For this review, take the finished solid that the model builds, in its own axes (mm). A direction names the side the tool comes from. Coordinates: 2 decimals unless noted, no trailing zeros. Loops run counter-clockwise (first coordinate to the right, second up) from the corner with the lowest first, then second, coordinate; pieces in that order, holes last. Notation, with made-up numbers: (12, 65.25) - (51, 65.25) arc R19 cw to (51, 69.25) - close; hole circle Ø7 at (19.5, -17). An arc over 180 degrees is marked (long way). Answer as a JSON object with one key per item and string values. Group by question number.
Item 1: We need section C-C (x = 3.25). Give the boundary of the cut face in (y, z).
Item 2: We need section A-A (x = -4.5). Give the boundary of the cut face in (y, z).
Item 3: Mouldability with a two-part tool opening along Z and no side actions: class faces 4 (the cylindrical face through (0.01, -7.985, -5.301)), 5 (the flat face through (-4, -2, -5)), 6 (the flat face through (-4, -6, 3)), 7 (the flat face through (0, -5, -2)) as released by +Z, released by -Z, zero draft, split by the parting line, or undercut.
Item 4: We need section B-B (y = 2.5). Give the boundary of the cut face in (x, z).
Item 5: Clearance check with flat-ended pins moving along their axes: pin 1 (6 mm diameter, centred on x = -2.5, z = -1.5, fed in from -Y); pin 2 (1.2 mm diameter, centred on x = -4, y = -7.5, fed in from +Z); pin 3 (1.3 mm diameter, centred on y = 0, z = 5, fed in from -X); pin 4 (1.5 mm diameter, centred on x = 3.5, z = 4, fed in from -Y). State where each tip first meets the part, or that it passes through.
Item 6: To check wall thickness, follow line 1 (Y direction, x = -5, z = 0.5); line 2 (X direction, y = -2.5, z = 4.25); line 3 (Z direction, x = 5.5, y = 2.75). State the ranges of each line that lie inside material, in increasing order.
Item 7: Tool access review of faces 1 (the cylindrical face through (-4.077, -10.416, -0.314)), 2 (the conical face through (-0.297, -0.904, 4.867)), 3 (the flat face through (4, -6, 3)): name each direction out of +Z, -Z, +X, -X, +Y, -Y from which nothing blocks a thin tool from reaching the whole face with its end or side.
from build123d import *

# Parameters (mm, degrees)
BOSS_EXTRUDE1_DEPTH      = 5
CUT_EXTRUDE8_DEPTH       = 10.848857802
CUT_EXTRUDE8_DEPTH_BACK  = 10.848857802
REVOLVE1_ANGLE           = 180
SKETCH24_W               = 3.9
SKETCH24_H               = 6
BOSS_EXTRUDE2_DEPTH      = 4
SKETCH25_W               = 3.9
SKETCH25_H               = 3
REVOLVE2_ANGLE           = 180
SKETCH26_R               = 1.45
CUT_EXTRUDE9_DEPTH       = 19
BOSS_EXTRUDE4_DEPTH      = 3.7
CUT_EXTRUDE10_DEPTH      = 19
CUT_EXTRUDE10_DEPTH_BACK = 19


with BuildPart() as part:
    # Sketch2 → Boss-Extrude1 (new, symmetric)
    with BuildSketch(Plane(origin=(0, 0, 0), x_dir=(1, 0, 0), z_dir=(0, 1, 0))):
        Polygon((-3, 6), (3, 6), (6, 3), (6, -3), (3, -6), (-3, -6), (-6, -3), (-6, 3), align=None)
    extrude(amount=BOSS_EXTRUDE1_DEPTH, both=True)

    # Sketch22 → Cut-Extrude8 (cut, two sides: drawn at the far end of the back side and taken through both)
    with BuildSketch(Plane(origin=(0, 0, 0), x_dir=(0, 0, -1), z_dir=(1, 0, 0)).offset(-CUT_EXTRUDE8_DEPTH_BACK)):
        Polygon((0, -5), (-6, -5), (-6, -1.535898385), align=None)
    extrude(amount=CUT_EXTRUDE8_DEPTH + CUT_EXTRUDE8_DEPTH_BACK, mode=Mode.SUBTRACT)

    # Sketch23 → Revolve1 (revolve)
    with BuildSketch(Plane(origin=(0, 5, 0), x_dir=(1, 0, 0), z_dir=(0, 1, 0))):
        Polygon((-6, 0), (-6, 3), (-3, 6), (3, 6), (6, 3), (6, 0), align=None)
    revolve(axis=Axis((6, 5, 0), (1, 0, 0)), revolution_arc=REVOLVE1_ANGLE)

    # Sketch24 → Boss-Extrude2 (add, symmetric)
    with BuildSketch(Plane.XZ.offset(5)):
        with Locations((-4.05, 0)):
            Rectangle(SKETCH24_W, SKETCH24_H)
    boss_extrude2 = extrude(amount=BOSS_EXTRUDE2_DEPTH, both=True)

    # Sketch25 → Revolve2 (revolve)
    with BuildSketch(Plane.XZ.offset(9)):
        with Locations((-4.05, 1.5)):
            Rectangle(SKETCH25_W, SKETCH25_H)
    revolve2 = revolve(axis=Axis((-6, -9, 0), (1, 0, 0)), revolution_arc=REVOLVE2_ANGLE)

    # Sketch26 → Cut-Extrude9 (cut, symmetric)
    with BuildSketch(Plane.ZY.offset(6)):
        with Locations((0, -9)):
            Circle(SKETCH26_R)
    cut_extrude9 = extrude(amount=CUT_EXTRUDE9_DEPTH, both=True, mode=Mode.SUBTRACT)

    # Mirror1: Boss-Extrude2, Revolve2, Cut-Extrude9 across plane
    add(boss_extrude2.mirror(Plane(origin=(0, 0, 0), x_dir=(0, 0, 1), z_dir=(1, 0, 0))))
    add(revolve2.mirror(Plane(origin=(0, 0, 0), x_dir=(0, 0, 1), z_dir=(1, 0, 0))))
    add(cut_extrude9.mirror(Plane(origin=(0, 0, 0), x_dir=(0, 0, 1), z_dir=(1, 0, 0))), mode=Mode.SUBTRACT)

    # Sketch30 → Cut-Revolve1 (revolve, cut)
    with BuildSketch(Plane(origin=(0, -3.75, 2.165063509), x_dir=(1, 0, 0), z_dir=(0, -0.8660254037844418, 0.49999999999999484))):
        Polygon((0, 3.42820323), (-0.75, 2.67820323), (-0.75, 1.92820323), (0.75, 1.92820323), (0.75, 2.67820323), align=None)
    revolve(axis=Axis((-6, -1.535898385, 6), (1, 0, 0)), mode=Mode.SUBTRACT)

    # Sketch34 → Boss-Extrude4 (add)
    with BuildSketch(Plane.XZ.offset(5)):
        Polygon((-6, -3), (-2.1, -3), (2.1, -3), (6, -3), (3, -6), (-3, -6), align=None)
    extrude(amount=BOSS_EXTRUDE4_DEPTH)

    # Sketch35 → Cut-Revolve3 (revolve, cut)
    with BuildSketch(Plane.XZ.offset(8.7)):
        Polygon((0, -3.5), (-0.75, -4.25), (-0.75, -5), (0.75, -5), (0.75, -4.25), align=None)
    revolve(axis=Axis((3, -8.7, -6), (1, 0, 0)), mode=Mode.SUBTRACT)

    # Sketch36 → Cut-Extrude10 (cut, two sides: drawn at the far end of the back side and taken through both)
    with BuildSketch(Plane.ZY.offset(6).offset(-CUT_EXTRUDE10_DEPTH_BACK)):
        Polygon((-3, -9), (0, -12), (0, -13.528535059), (-3.643435522, -13.528535059), (-3.643435522, -9), align=None)
    extrude(amount=CUT_EXTRUDE10_DEPTH + CUT_EXTRUDE10_DEPTH_BACK, mode=Mode.SUBTRACT)


solid = part.part
Check sheet entries:
{
 "1": {"outline": "(-12, 0) - (-9, -3) - (-8.7, -3) - (-8.7, -5.75) - (5, -5.75) arc R5.75 ccw to (5, 5.75) - (-1.68, 5.75) - (-3.27, 3) - (-9, 3) arc R3 ccw to start; hole circle Ø2.9 at (-9, 0)"},
 "2": {"outline": "(-12, 0) - (-9, -3) - (-8.7, -3) - (-8.7, -4.5) - (5, -4.5) arc R4.5 ccw to (5, 4.5) - (-2.4, 4.5) - (-3.27, 3) - (-9, 3) arc R3 ccw to start; hole circle Ø2.9 at (-9, 0)"},
 "3": {"face 4": "undercut", "face 5": "released by -Z", "face 6": "released by +Z", "face 7": "zero draft"},
 "4": {"outline": "(-6, -3) - (-3, -6) - (3, -6) - (6, -3) - (6, 3) - (3, 6) - (-3, 6) - (-6, 3) - close"},
 "5": {"pin 1": "stops at y = -12", "pin 2": "stops at z = 3", "pin 3": "stops at x = -4.65", "pin 4": "stops at y = -3.12"},
 "6": {"line 1": "y = -11.96 to -10.36, -7.64 to 8.97", "line 2": "x = -4.75 to -0.75, 0.75 to 4.75", "line 3": "z = -3.5 to 3.5"},
 "7": {"face 1": "+X, -X", "face 2": "none", "face 3": "+Z, +X, -X, -Y"}
}
